Could you check a few things on this model? Use its own coordinates, in mm. A direction names the side the tool comes from. Coordinates: 2 decimals unless noted, no trailing zeros. Loops run counter-clockwise (first coordinate to the right, second up) from the corner with the lowest first, then second, coordinate; pieces in that order, holes last. Notation, with made-up numbers: (82, 63.5) - (115, 63.5) arc R38 ccw to (115, 101.5) - close; hole circle Ø7 at (34, 16.5). An arc over 180 degrees is marked (long way). One line per question, with ' | ' between items. Start each with the question number.
1. Which directions (+Z, -Z, +X, -X, +Y, -Y) give clear straight access to the entire face, cutting with the end or side of a thin tool? Please do faces 1 (the flat face through (89, 2, -90)), 2 (the flat face through (112, 2, -45)).
2. I want a section at A-A, the plane x = 70. Write out the boundary of the cut face in (y, z).
3. I want a section at C-C, the plane y = 1.15. Count the separate pieces of the cut face and the enclosed holes in it, then the cut area to 3 significant figures.
4. Please list where these lines run through material, in increasing order: L1, parallel to X at y = 2.05, z = -35.5; L2, parallel to Z at x = 170.5, y = 1.35; L3, parallel to X at y = 1.6, z = -84. Write a range as [from, to].
5. I want a section at B-B, the plane z = -38. Write out the boundary of the cut face in (x, y), then the cut area to 3 significant figures.
6. I'm going to push a flat-ended pin straight in: P1, Ø3, axis at x = 144.5, z = -58, coming from the +Y side. Where does the tip first touch, or does it pass through?
from build123d import *

# Parameters (mm, degrees)
SKETCH_1_W      = 180
SKETCH_1_H      = 90
SKETCH_1_R      = 1.55
EXTRUDE_1_DEPTH = 4
SKETCH_3_W      = 90
SKETCH_3_H      = 4
EXTRUDE_2_DEPTH = 5
SKETCH_4_W      = 90
SKETCH_4_H      = 4
EXTRUDE_3_DEPTH = 5


with BuildPart() as part:
    # 草图1 → 凸台-拉伸1 (new body)
    with BuildSketch(Plane(origin=(0, 0, 0), x_dir=(1, 0, 0), z_dir=(0, 1, 0))):
        with Locations((90, 45)):
            Rectangle(SKETCH_1_W, SKETCH_1_H)
        with Locations(Location((9.5, 58, 0), (0, 0, 270))):
            Circle(SKETCH_1_R, mode=Mode.SUBTRACT)
        with Locations(Location((35.5, 58, 0), (0, 0, 270))):
            Circle(SKETCH_1_R, mode=Mode.SUBTRACT)
        with Locations(Location((35.5, 32, 0), (0, 0, 270))):
            Circle(SKETCH_1_R, mode=Mode.SUBTRACT)
        with Locations(Location((9.5, 32, 0), (0, 0, 270))):
            Circle(SKETCH_1_R, mode=Mode.SUBTRACT)
        with Locations(Location((144.5, 58, 0), (0, 0, 90))):
            Circle(SKETCH_1_R, mode=Mode.SUBTRACT)
        with Locations(Location((170.5, 58, 0), (0, 0, 90))):
            Circle(SKETCH_1_R, mode=Mode.SUBTRACT)
        with Locations(Location((170.5, 32, 0), (0, 0, 90))):
            Circle(SKETCH_1_R, mode=Mode.SUBTRACT)
        with Locations(Location((144.5, 32, 0), (0, 0, 90))):
            Circle(SKETCH_1_R, mode=Mode.SUBTRACT)
        with Locations(Location((127.9, 58, 0), (0, 0, 270))):
            Circle(SKETCH_1_R, mode=Mode.SUBTRACT)
        with Locations(Location((174, 84, 0), (0, 0, 270))):
            Circle(SKETCH_1_R, mode=Mode.SUBTRACT)
        with Locations(Location((174, 6, 0), (0, 0, 90))):
            Circle(SKETCH_1_R, mode=Mode.SUBTRACT)
        with Locations(Location((6, 6, 0), (0, 0, 270))):
            Circle(SKETCH_1_R, mode=Mode.SUBTRACT)
        with Locations(Location((6, 84, 0), (0, 0, 90))):
            Circle(SKETCH_1_R, mode=Mode.SUBTRACT)
        with Locations(Location((52.1, 58, 0), (0, 0, 90))):
            Circle(SKETCH_1_R, mode=Mode.SUBTRACT)
        with Locations(Location((127.9, 32, 0), (0, 0, 90))):
            Circle(SKETCH_1_R, mode=Mode.SUBTRACT)
        with Locations(Location((52.1, 32, 0), (0, 0, 270))):
            Circle(SKETCH_1_R, mode=Mode.SUBTRACT)
        with BuildLine():
            Line((68, 35), (68, 55))
            ThreePointArc((68, 55), (70, 57), (72, 55))
            Line((72, 55), (72, 35))
            ThreePointArc((72, 35), (70, 33), (68, 35))
        make_face(mode=Mode.SUBTRACT)
        with BuildLine():
            Line((112, 35), (112, 55))
            ThreePointArc((112, 55), (110, 57), (108, 55))
            Line((108, 55), (108, 35))
            ThreePointArc((108, 35), (110, 33), (112, 35))
        make_face(mode=Mode.SUBTRACT)
    extrude(amount=EXTRUDE_1_DEPTH)

    # 草图3 → 凸台-拉伸2 (add)
    with BuildSketch(Plane.ZY):
        with Locations((-45, 2)):
            Rectangle(SKETCH_3_W, SKETCH_3_H)
    extrude(amount=EXTRUDE_2_DEPTH)

    # 草图4 → 凸台-拉伸3 (add)
    with BuildSketch(Plane(origin=(180, 0, 0), x_dir=(0, 0, -1), z_dir=(1, 0, 0))):
        with Locations((45, 2)):
            Rectangle(SKETCH_4_W, SKETCH_4_H)
    extrude(amount=EXTRUDE_3_DEPTH)


solid = part.part
Results are:
1) face 1: -Z, +X, -X, +Y, -Y | face 2: +Y, -Y
2) outline: (0, -90) - (4, -90) - (4, -57) - (0, -57) - close; (0, -33) - (4, -33) - (4, 0) - (0, 0) - close
3) separate pieces: 1 | enclosed holes: 18 | area: 16,800 mm2
4) L1: x = [-5, 68], [72, 108], [112, 185] | L2: z = [-90, -59.55], [-56.45, -33.55], [-30.45, 0] | L3: x = [-5, 4.45], [7.55, 172.45], [175.55, 185]
5) outline: (-5, 0) - (68, 0) - (68, 4) - (-5, 4) - close; (72, 0) - (108, 0) - (108, 4) - (72, 4) - close; (112, 0) - (185, 0) - (185, 4) - (112, 4) - close | area: 728 mm2
6) P1: passes through
